Design review of the part shown in the three views and the two pictorial views. Dimensions are in mm from the part's minimum x, y and z. Round coordinates to 2 decimals unless told otherwise and drop trailing zeros. Loops run counter-clockwise (first coordinate to the right, second up) from the corner with the lowest first, then second, coordinate; pieces in that order, holes last. Notation, with made-up numbers: (77, -11) - (94, -11) arc R28 ccw to (94, 15) - close; hole circle Ø8 at (-1.75, 6). An arc over 180 degrees is marked (long way). Return JSON: item names as keys, results as strings. Group by question number.
(1) Wall thickness on L1, parallel to Z at x = 6.25, y = 4; L2, parallel to Y at x = 5.25, z = 13 (1 decimal); L3, parallel to X at y = 6.25, z = 4.25 (1 decimal): over which ranges is each line inside the solid? List them lowest first. Write a range as [from, to].
(2) We need section B-B, the plane x = 4. Write out the cut boundary in (y, z).
(3) The part is to be moulded in two halves that separate along Y. For the marked faces 1 and 2, say which applies: pulls with the +Y half, pulls with the -Y half, needs draft (parallel to the pull), parting line crosses it, or undercut.
(4) We need section C-C, the plane z = 2.75. Write out the cut boundary in (x, y) (1 decimal).
(5) Clearance check with flat-ended pins moving along their axes: pin 1 (4 mm diameter, centred on x = 5, z = 7.5, fed in from +Y) (1 decimal); pin 2 (1 mm diameter, centred on y = 6, z = 17, fed in from +X); pin 3 (4 mm diameter, centred on x = 4.76, y = 4.76, fed in from -Z). State where each tip first meets the part, or that it passes through.
(6) We need section D-D, the plane x = 7.75. Write out the cut boundary in (y, z).
(7) We need section A-A, the plane y = 2.75. Write out the cut boundary in (x, z), and give its area (3 significant figures).
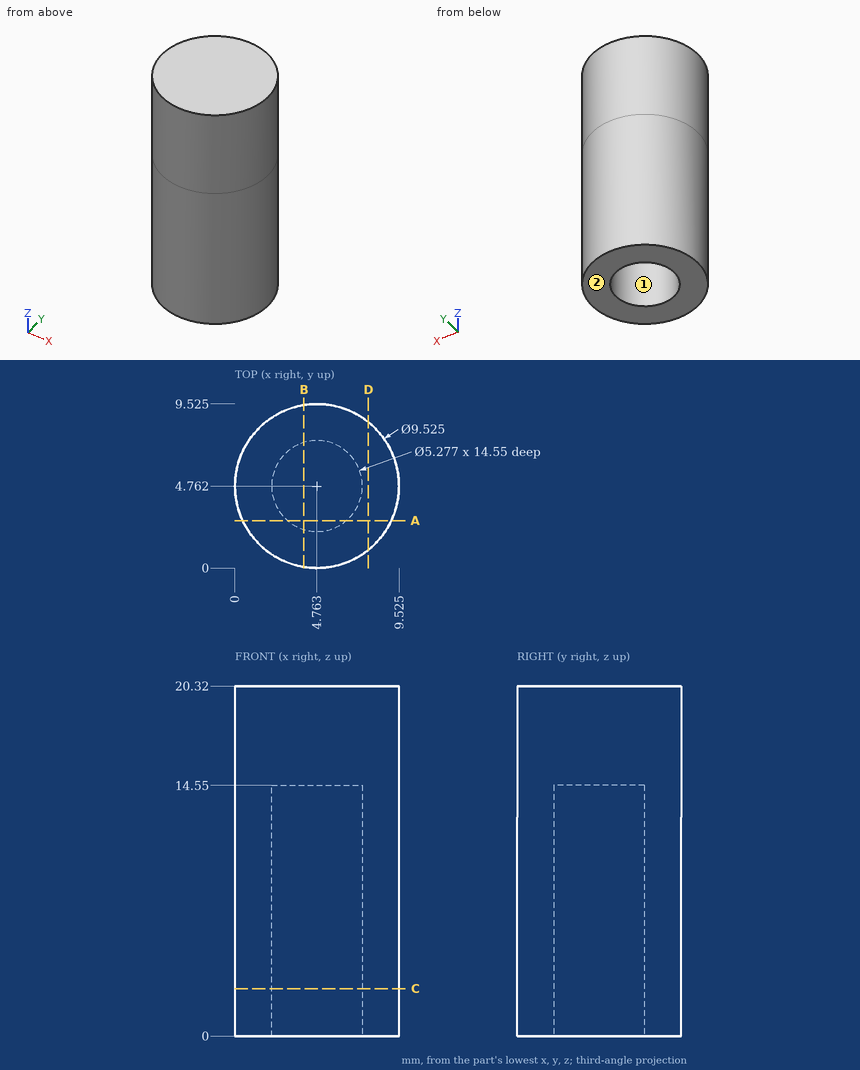
Solutions:
{
 "1": {"L1": "[14.55, 20.32]", "L2": "[0, 2.2], [7.4, 9.5]", "L3": "[0.2, 2.6], [6.9, 9.3]"},
 "2": {"outline": "(0.06, 0) - (2.24, 0) - (2.24, 14.55) - (7.29, 14.55) - (7.29, 0) - (9.46, 0) - (9.46, 20.32) - (0.06, 20.32) - close"},
 "3": {"face 1": "undercut", "face 2": "needs draft"},
 "4": {"outline": "circle Ø9.5 at (4.8, 4.8); hole circle Ø5.3 at (4.8, 4.8)"},
 "5": {"pin 1": "y = 9.5", "pin 2": "x = 9.47", "pin 3": "z = 14.55"},
 "6": {"outline": "(1.05, 0) - (8.47, 0) - (8.47, 20.32) - (1.05, 20.32) - close"},
 "7": {"outline": "(0.45, 0) - (3.06, 0) - (3.06, 14.55) - (6.47, 14.55) - (6.47, 0) - (9.08, 0) - (9.08, 20.32) - (0.45, 20.32) - close", "area": "126 mm^2"}
}
